Could you check a few things on this model? Use its own coordinates, in mm. A direction names the side the tool comes from. Coordinates: 2 decimals unless noted, no trailing zeros. Order: outer loops, then holes, each group sorted by start corner. A loop starts at its lowest first (then second) coordinate and runs counter-clockwise, first axis right, second up. Notation, with made-up numbers: M 26.25,87 L 41.25,87 A18 cw 41.25,112 Z; hole C 0,20 d6. An arc over 180 degrees is marked long. Write item = value, one per line. Start each with the question number.
from build123d import *

# Parameters (mm, degrees)
F0_R      = 25.4
F1_DEPTH  = 3.175
F2_R      = 3.175
F3_DEPTH  = 76.2
F5_DEPTH  = 3.175
F7_DEPTH  = 3.175
F9_DEPTH  = 76.2
F10_W     = 12.8941143926
F10_H     = 3.6661742094
F11_DEPTH = 50.8
F12_W     = 7.7148651539
F12_H     = 3.6661742094
F13_DEPTH = 25.4


with BuildPart() as f1:
    # F0 (on Top) → F1 (new body)
    with BuildSketch(Plane.XY):
        Circle(F0_R)
    extrude(amount=F1_DEPTH)

    # F2 (on face) → F3 (join)
    with BuildSketch(Plane.XY.offset(3.175)):
        Circle(F2_R)
    extrude(amount=F3_DEPTH)

    # F4 (on Top) → F5 (join)
    with BuildSketch(Plane.XY):
        Polygon((-24.8449490586, 5.2809569468), (-24.2898981173, 0), (-23.2040546241, -10.3311107341), (-12.7, -21.9970452561), (2.655022967, -25.2608561424), (16.9959174015, -18.8758785671), (24.8449490586, -5.2809569468), (23.2040546241, 10.3311107341), (12.7, 21.9970452561), (-2.655022967, 25.2608561424), (-16.9959174015, 18.8758785671), align=None)
    extrude(amount=-F5_DEPTH)

    # F6 (on face) → F7 (join)
    with BuildSketch(Plane(origin=(17.9520273121, 16.1640779951, 0), x_dir=(-0.6691306064, 0.7431448255, 0), z_dir=(0.7431448255, 0.6691306064, 0))):
        Polygon((22.7787770654, -4.8509683429), (7.8490316571, 0), (-7.0807137511, -4.8509683429), (-16.3078038568, -17.5509683429), (-16.3078038568, -33.2490316571), (-7.0807137511, -45.9490316571), (7.8490316571, -50.8), (22.7787770654, -45.9490316571), (32.005867171, -33.2490316571), (32.005867171, -17.5509683429), align=None)
    extrude(amount=F7_DEPTH)

    # F8 (on face) → F9 (join)
    with BuildSketch(Plane(origin=(20.311512133, 18.2885676703, 0), x_dir=(-0.6691306064, 0.7431448255, 0), z_dir=(0.7431448255, 0.6691306064, 0))):
        Polygon((11.0240316571, -27.2330871047), (11.0240316571, -23.5669128953), (7.8490316571, -21.7338257906), (4.6740316571, -23.5669128953), (4.6740316571, -27.2330871047), (7.8490316571, -29.0661742094), align=None)
    extrude(amount=F9_DEPTH)

    # F10 (on face) → F11 (join)
    with BuildSketch(Plane(origin=(-3.1275376369, 3.4734824401, 0), x_dir=(0.7431448255, 0.6691306064, 0), z_dir=(0.6691306064, -0.7431448255, 0))):
        with Locations((97.0847783176, -25.4)):
            Rectangle(F10_W, F10_H)
    extrude(amount=F11_DEPTH)

    # F12 (on face) → F13 (join)
    with BuildSketch(Plane(origin=(76.9391478343, 69.2763198749, 0), x_dir=(-0.6691306064, 0.7431448255, 0), z_dir=(0.7431448255, 0.6691306064, 0))):
        with Locations((-42.2685357659, -25.4)):
            Rectangle(F12_W, F12_H)
    extrude(amount=F13_DEPTH)


solid = f1.part
(1) Imagine slicing it at C-C on x = 34. List the corners of the cut face in (y, z) for me.
(2) Imagine slicing it at A-A on y = 49.5. List the corners of the cut face in (x, z) for me.
(3) Will these pins go through, and if not, where does the flat tip stop? P1, Ø3.5, axis at x = -6.5, y = -24, coming from the -Z side (3 decimals); P2, Ø12, axis at x = 58, y = 55.5, coming from the -Z side; P3, Ø5, axis at x = 94.5, y = 32, coming from the +Z side; P4, Ø1.9, axis at x = 13, y = -23, coming from the -Z side.
(4) Please list where these lines run through material, in increasing order: probe 1 along Z at (x, y) = (5.5, 19) (3 decimals); probe 2 along X at (y, z) = (-0.5, 71.5); probe 3 along X at (y, z) = (61.5, -26). Write a range as from..to.
(5) Imagine slicing it at B-B on z = 27.5. List the corners of the cut face in (x, y) for me (3 decimals).
(6) Thinking about a two-plate mould opening in Z: for faces 1 (the flat face through (112.25, 39, -25.43)), 2 (the flat face through (44.054, 48.062, -28.137)), 3 (the flat face through (19, 15, -1)), which applies, released by +Z, released by -Z, zero draft, split by the parting line, or undercut?
(7) For faces 4 (the flat face through (-9.73, 22.11, -1.57)), 5 (the flat face through (9.73, -22.11, -1.57)), 6 (the flat face through (0, 0, -3.175)), 7 (the cylindrical face through (-0.69, -3.1, 40.74)), 8 (the flat face through (41.9, 50.45, -22.66)), which set-ups out of +Z, -Z, +X, -X, +Y, -Y let a thin tool reach every point of the face, with its end or its side?
(8) Imagine slicing it at D-D on x = 91. List the corners of the cut face in (y, z) for me, plus the area to 3 significant figures.
Response:
q1.outline = M 36.9,-27.23 L 41.18,-29.07 L 45.45,-27.23 L 45.45,-23.57 L 41.18,-21.73 L 36.9,-23.57 Z
q2.outline = M 38.5,-27.23 L 43.25,-29.07 L 47.99,-27.23 L 47.99,-23.57 L 43.25,-21.73 L 38.5,-23.57 Z; M 77.4,-27.23 L 94.75,-27.23 L 94.75,-23.57 L 77.4,-23.57 Z; M 112.38,-27.23 L 123.91,-27.23 L 123.91,-23.57 L 112.38,-23.57 Z
q3.P1 = -3.175
q3.P2 = -29.07
q3.P3 = -23.57
q3.P4 = through
q4.probe_1 = -3.175..3.175
q4.probe_2 = -3.14..3.14
q4.probe_3 = 51.83..61.32, 66.59..83.94
q5.outline = C 0,0 d6.35
q6.face_1 = zero draft
q6.face_2 = released by -Z
q6.face_3 = undercut
q7.face_4 = -Z, -X, +Y
q7.face_5 = -Z, +X, -Y
q7.face_6 = -Z, -X, -Y
q7.face_7 = +Z
q7.face_8 = +Z, +Y
q8.outline = M 34.39,-27.23 L 53.66,-27.23 L 53.66,-23.57 L 34.39,-23.57 Z
q8.area = 70.6 mm2
